Verification items for the finished model (mm, model axes). A direction names the side the tool comes from. Coordinates: 2 decimals unless noted, no trailing zeros. Order: outer loops, then holes, each group sorted by start corner. A loop starts at its lowest first (then second) coordinate and runs counter-clockwise, first axis right, second up. Notation, with made-up numbers: M 37.5,-4 L 51.5,-4 A12 ccw 51.5,10 Z; hole C -9,71.5 d11. An arc over 180 degrees is marked long. Return JSON: item names as keys, results as strings. Group by question number.
1. Mould release check, pull along Z, two halves, no side actions. Record for faces 4 (the flat face through (0, 0, 1.3)), 5 (the cylindrical face through (0.355, -0.634, 2.855)), 6 (the flat face through (0.74, -0.87, 0.49)): +Z half, -Z half, draft (parallel to the pull), parting line (faces both ways), or undercut.
2. Section check A-A, the plane y = 0. Record the cut outline in (x, z) (3 decimals).
3. Gauge pin test, flat ends, axial feed: pin 1 (1 mm diameter, centred on x = 6, z = 0, fed in from +Y); pin 2 (1.5 mm diameter, centred on x = 1.5, z = -1.5, fed in from +Y); pin 3 (2 mm diameter, centred on x = 1, z = 1.5, fed in from +Y). Record the tip position at first contact, or that the pin passes through.
4. Section check C-C, the plane x = 4. Record the cut outline in (y, z).
5. Material ranges on line 1 along X through (y, z) = (-0.45, 0.5); line 2 along X through (y, z) = (-1.65, -1.9); line 3 along Y through (x, z) = (1, -0.65), recorded low to high.
6. Set-up check for faces 1 (the flat face through (8, 0, 0)), 2 (the flat face through (1, 0, -1)), 3 (the cylindrical face through (5.18, -1.45, -0.06)): record each of +Z, -Z, +X, -X, +Y, -Y from which the full face is reachable in a straight line by a thin tool's end or side.
7. Section check B-B, the plane x = 1.25. Record the cut outline in (y, z).
```python
from build123d import *

# Parameters (mm, degrees)
CUT_EXTRUDE1_DEPTH = 1.5


with BuildPart() as part:
    # Sketch1 → Revolve1 (revolve)
    with BuildSketch(Plane.XY):
        with BuildLine():
            Line((2.534073147, 1.45), (7.752512627, 1.45))
            Line((7.752512627, 1.45), (8, 1.202512627))
            Line((8, 1.202512627), (8, 0))
            Line((8, 0), (0, 0))
            Line((0, 0), (0, 2.925))
            Line((0, 2.925), (0.7, 2.925))
            Line((0.7, 2.925), (2.2, 1.577985037))
            ThreePointArc((2.2, 1.577985037), (2.355198165, 1.483091293), (2.534073147, 1.45))
        make_face()
    revolve(axis=Axis((0, 0, 0), (-1, 0, 0)))

    # Sketch2 → Cut-Extrude1 (cut)
    with BuildSketch(Plane.ZY):
        Polygon((1, 0.577350269), (0, 1.154700538), (-1, 0.577350269), (-1, -0.577350269), (0, -1.154700538), (1, -0.577350269), align=None)
    extrude(amount=-CUT_EXTRUDE1_DEPTH, mode=Mode.SUBTRACT)


solid = part.part
```
Answers follow:
{
 "1": {"face 4": "draft", "face 5": "parting line", "face 6": "undercut"},
 "2": {"outline": "M 0,-2.925 L 0.7,-2.925 L 2.2,-1.578 A0.5 cw 2.534,-1.45 L 7.753,-1.45 L 8,-1.203 L 8,1.203 L 7.753,1.45 L 2.534,1.45 A0.5 cw 2.2,1.578 L 0.7,2.925 L 0,2.925 L 0,1 L 1.5,1 L 1.5,-1 L 0,-1 Z"},
 "3": {"pin 1": "y = 1.45", "pin 2": "y = 2.56", "pin 3": "y = 2.87"},
 "4": {"outline": "C 0,0 d2.9"},
 "5": {"line 1": "1.5 to 8", "line 2": "0 to 1.15", "line 3": "-2.57 to -0.78, 0.78 to 2.57"},
 "6": {"face 1": "+Z, -Z, +X, +Y, -Y", "face 2": "-X", "face 3": "+X"},
 "7": {"outline": "C 0,0 d4.86; hole M -1.15,0 L -0.58,-1 L 0.58,-1 L 1.15,0 L 0.58,1 L -0.58,1 Z"}
}
